```python
from build123d import *

# Parameters (mm, degrees)
SKIZZE1_W                       = 36
SKIZZE1_H                       = 30
AUFSATZ_LINEAR_AUSTRAGEN1_DEPTH = 4
SKIZZE2_R                       = 5.5
SKIZZE2_R_2                     = 0.875
SCHNITT_LINEAR_AUSTRAGEN1_DEPTH = 4
SKIZZE3_W                       = 4
SKIZZE3_H                       = 10
SKIZZE3_W_2                     = 10
SKIZZE3_H_2                     = 4
SCHNITT_LINEAR_AUSTRAGEN2_DEPTH = 24.769728648


with BuildPart() as part:
    # Skizze1 → Aufsatz-Linear austragen1 (new body)
    with BuildSketch(Plane.XY):
        Rectangle(SKIZZE1_W, SKIZZE1_H)
    extrude(amount=AUFSATZ_LINEAR_AUSTRAGEN1_DEPTH)

    # Skizze2 → Schnitt-Linear austragen1 (cut)
    with BuildSketch(Plane.XY.offset(4)):
        Circle(SKIZZE2_R)
        with Locations((5.656854249, 5.656854249)):
            Circle(SKIZZE2_R_2)
        with Locations((6.363961031, -6.363961031)):
            Circle(SKIZZE2_R_2)
        with Locations(Location((-5.656854249, -5.656854249, 0), (0, 0, 180))):
            Circle(SKIZZE2_R_2)
        with Locations(Location((-6.363961031, 6.363961031, 0), (0, 0, 180))):
            Circle(SKIZZE2_R_2)
    extrude(amount=-SCHNITT_LINEAR_AUSTRAGEN1_DEPTH, mode=Mode.SUBTRACT)

    # Skizze3 → Schnitt-Linear austragen2 (cut, through all)
    with BuildSketch(Plane.XY.offset(4)):
        with Locations((-16, 0)):
            Rectangle(SKIZZE3_W, SKIZZE3_H)
        with Locations((0, 13)):
            Rectangle(SKIZZE3_W_2, SKIZZE3_H_2)
        with Locations((16, 0)):
            Rectangle(SKIZZE3_W, SKIZZE3_H)
    extrude(amount=-SCHNITT_LINEAR_AUSTRAGEN2_DEPTH, mode=Mode.SUBTRACT)


solid = part.part
```
Could you check a few things on this model? Use its own coordinates, in mm. A direction names the side the tool comes from. Round coordinates to 2 decimals unless told otherwise and drop trailing zeros. Loops run counter-clockwise (first coordinate to the right, second up) from the corner with the lowest first, then second, coordinate; pieces in that order, holes last.
Q1. Please list where these lines run through material, in increasing order: L1, parallel to X at y = 13.5, z = 3.15; L2, parallel to Y at x = 16, z = 1.5; L3, parallel to Y at x = 0, z = 2.3.
Q2. I want a section at C-C (z = 1.6). Write out the boundary of the cut face in (x, y) (3 decimals), and give its area (3 significant figures).
Q3. For P1, Ø2, axis at y = 2, z = 2.5, coming from the +X side; P2, Ø2, axis at y = -0.5, z = 2, coming from the -X side, each with a flat end and sliding along its axis, tell me the tip position at first contact or that it passes through.
Q4. Thinking about a two-plate mould opening in X: for faces 1 (the cylindrical face through (5.012, 6.248, 2.028)), 2 (the flat face through (14, 0, 2)), 3 (the flat face through (11, 15, 2)), 4 (the flat face through (5, 13, 2)), which applies, pulls with the +X half, pulls with the -X half, needs draft (parallel to the pull), parting line crosses it, or undercut?
Q5. On a 3-axis mill with a long thin cutter (end or side, diameter ignored), from which of +Z, -Z, +X, -X, +Y, -Y can I reach the whole of each face in a straight line? I mean faces 5 (the flat face through (0, 11, 2)), 6 (the cylindrical face through (-6.25, 5.496, 2.028)), 7 (the flat face through (-18, -10, 2)), 8 (the flat face through (-14, 0, 2)), 9 (the flat face through (16, -5, 2)). Say none if no direction works.
Q6. I want a section at A-A (x = 16). Write out the boundary of the cut face in (y, z), and give its area (3 significant figures).
Q7. I want a section at B-B (y = 0). Write out the boundary of the cut face in (x, z).
Answer below:
1. L1: x = -18 to -5, 5 to 18
1. L2: y = -15 to -5, 5 to 15
1. L3: y = -15 to -5.5, 5.5 to 11
2. outline: (-18, -15) - (18, -15) - (18, -5) - (14, -5) - (14, 5) - (18, 5) - (18, 15) - (5, 15) - (5, 11) - (-5, 11) - (-5, 15) - (-18, 15) - (-18, 5) - (-14, 5) - (-14, -5) - (-18, -5) - close; hole circle Ø1.75 at (-6.364, 6.364); hole circle Ø1.75 at (-5.657, -5.657); hole circle Ø11 at (0, 0); hole circle Ø1.75 at (5.657, 5.657); hole circle Ø1.75 at (6.364, -6.364)
2. area: 855 mm2
3. P1: stops at x = 14
3. P2: stops at x = -14
4. face 1: undercut
4. face 2: pulls with the +X half
4. face 3: needs draft
4. face 4: undercut
5. face 5: +Z, -Z, +Y
5. face 6: +Z, -Z
5. face 7: +Z, -Z, -X, +Y, -Y
5. face 8: +Z, -Z, -X
5. face 9: +Z, -Z, +X
6. outline: (-15, 0) - (-5, 0) - (-5, 4) - (-15, 4) - close; (5, 0) - (15, 0) - (15, 4) - (5, 4) - close
6. area: 80.0 mm2
7. outline: (-14, 0) - (-5.5, 0) - (-5.5, 4) - (-14, 4) - close; (5.5, 0) - (14, 0) - (14, 4) - (5.5, 4) - close
